Autodesk Inventor part; units mm, degrees
ref_plane "YZ Plane" through (0, 0, 0) normal (1, 0, 0) x (0, 1, 0)
ref_plane "XZ Plane" through (0, 0, 0) normal (0, 1, 0) x (-1, 0, 0)
ref_plane "XY Plane" through (0, 0, 0) normal (0, 0, 1) x (1, 0, 0)
sketch "スケッチ1" plane through (0, 0, 0) normal (0, 1, 0) x (-1, 0, 0)
  circle A0 centre (0, 0) radius 65
  circle A1 centre (0, 0) radius 60
  circle A2 centre (0, 0) radius 16
  circle A3 centre (0, 0) radius 11
  dimension "d0" = 130
  dimension "d3" = 120
  dimension "d4" = 32
  dimension "d5" = 22
extrude "押し出し1" add sketch "スケッチ1" along normal blind 25 contours A0 | A1 | A2 | A3
extrude "押し出し2" cut sketch "スケッチ1" along normal blind 20 contours A1
extrude "押し出し3" cut sketch "スケッチ1" along normal blind 9 contours A3
properties part number "18-1"
Model file for the job. Use its own axes, mm. A direction names the side the tool comes from. Round coordinates to 2 decimals unless told otherwise and drop trailing zeros. Order: outer loops, then holes, each group sorted by start corner. A loop starts at its lowest first (then second) coordinate and runs counter-clockwise, first axis right, second up.
(1) Band-saw the part on B-B (x = 0). List the corners of the cut face in (y, z).
(2) Pull direction Z, two halves, no side cores. Call faces 1 (the face through (-12, 20, -12)), 2 (the face through (-62, 12.32, -19.52)), 3 (the face through (-3, 0, 11)): released by +Z, released by -Z, zero draft, split by the parting line, or undercut.
(3) Band-saw the part on C-C (y = 15.75). List the corners of the cut face in (x, z).
(4) Band-saw the part on D-D (z = 0). List the corners of the cut face in (x, y).
(5) 3-axis set-ups, long thin cutter, end or side, ignore diameter. For faces 4 (the face through (59.94, 9.86, -2.64)), 5 (the face through (1, 25, 1)): which of +Z, -Z, +X, -X, +Y, -Y reach the whole face in a straight line?
(6) Drill centre lines: line 1 (Z direction, x = 0, y = 5.5); line 2 (Z direction, x = 0, y = 12); line 3 (Z direction, x = 9.5, y = 14). Where is each one in solid material? Low to high.
(7) Pin check, flat tips, straight feed: pin 1 (6 mm diameter, centred on x = -25, z = -28, fed in from -Y); pin 2 (6.5 mm diameter, centred on x = -1.5, z = 5.5, fed in from -Y); pin 3 (1 mm diameter, centred on y = 9.5, z = 20.5, fed in from -X). Stop position of each tip, or through.
(8) Band-saw the part on A-A (y = 4.75). List the corners of the cut face in (x, z), then the cut area to 3 significant figures.
Verdict:
1. outline: (0, -65) - (25, -65) - (25, 65) - (0, 65) - (0, 60) - (20, 60) - (20, 16) - (0, 16) - (0, 11) - (9, 11) - (9, -11) - (0, -11) - (0, -16) - (20, -16) - (20, -60) - (0, -60) - close
2. face 1: undercut
2. face 2: split by the parting line
2. face 3: zero draft
3. outline: circle Ø130 at (0, 0); circle Ø32 at (0, 0); hole circle Ø120 at (0, 0)
4. outline: (-65, 0) - (-60, 0) - (-60, 20) - (-16, 20) - (-16, 0) - (-11, 0) - (-11, 9) - (11, 9) - (11, 0) - (16, 0) - (16, 20) - (60, 20) - (60, 0) - (65, 0) - (65, 25) - (-65, 25) - close
5. face 4: -Y
5. face 5: +Z, -Z, +X, -X, +Y
6. line 1: z = -65 to -60, -16 to -11, 11 to 16, 60 to 65
6. line 2: z = -65 to -60, -16 to 16, 60 to 65
6. line 3: z = -64.3 to -59.24, -12.87 to 12.87, 59.24 to 64.3
7. pin 1: stops at y = 20
7. pin 2: stops at y = 9
7. pin 3: stops at x = -61.85
8. outline: circle Ø130 at (0, 0); circle Ø32 at (0, 0); hole circle Ø120 at (0, 0); hole circle Ø22 at (0, 0)
8. area: 2,390 mm2
